Autodesk Inventor part; units mm, degrees
ref_plane "YZ Plane" through (0, 0, 0) normal (1, 0, 0) x (0, 1, 0)
ref_plane "XZ Plane" through (0, 0, 0) normal (0, 1, 0) x (-1, 0, 0)
ref_plane "XY Plane" through (0, 0, 0) normal (0, 0, 1) x (1, 0, 0)
sketch "Sketch1" plane through (0, 0, 0) normal (0, 1, 0) x (-1, 0, 0)
  line L0 (60, 25) -> (-60, 25)
  line L1 (-60, 25) -> (-60, -25)
  line L2 (-60, -25) -> (60, -25)
  line L3 (60, -25) -> (60, 25)
  point P0 (0, 0)
extrude "Extrusion1" add sketch "Sketch1" along normal mid plane 25
sketch "Sketch2" plane through (-60, 12.5, 25) normal (0, 0, 1) x (1, 0, 0)
  line L0 (0, -25) -> (120, -25)
  line L1 (60, -25) -> (20, -25)
  line L2 (20, -25) -> (20, -10)
  line L3 (20, -10) -> (100, -10)
  line L4 (100, -10) -> (100, -25)
  line L5 (100, -25) -> (60, -25)
  point P0 (60, -12.5)
  dimension "d5" = 15
  dimension "d6" = 80
extrude "Extrusion2" cut sketch "Sketch2" against normal through all
fillet "Fillet1" radius 12.5 2 edges at (60, 12.5, 0) (-60, 12.5, 0)
sketch "Sketch3" plane through (0, -12.5, 0) normal (0, -1, 0) x (1, 0, 0)
  line L0 (-60, 25) -> (-60, -25)
  line L1 (60, -25) -> (60, 25)
  point P0 (0, 0)
  point P1 (-50, 0)
  point P2 (50, 0)
hole "Hole1" at (-50, -12.5, 0) at (50, -12.5, 0) direction (0, 1, 0) diameter 3 depth 0.5 tip angle 118
properties part number "newsteelhandle" material "Steel"
Check sheet for the modelled part. Datum: model origin and axes. Units: mm. A direction names the side the tool comes from. Give positions to 0.01 mm unless a question says otherwise; leave off trailing zeros. Loops run counter-clockwise (first coordinate to the right, second up) from the corner with the lowest first, then second, coordinate; pieces in that order, holes last. Notation, with made-up numbers: M 34.5,-38 L 65.5,-38 A12 ccw 65.5,-24 Z; hole C -1,83.5 d8. An arc over 180 degrees is marked long. Return JSON: item names as keys, results as strings. Group by question number.
1. Mould release check, pull along X, two halves, no side actions. Record for faces 4 (the conical face through (50.078, -11.255, -0.248)), 5 (the cylindrical face through (56.241, 8.935, -0.35)), 6 (the flat face through (48, -12.5, 0)): released by +X, released by -X, zero draft, split by the parting line, or undercut.
2. Tool access check on faces 1 (the flat face through (-40, -5, 0)), 2 (the flat face through (60, -6, 0)), 3 (the cylindrical face through (51.464, -12.246, 0.325)). Record the directions out of +Z, -Z, +X, -X, +Y, -Y that give a thin tool (end or side, any length) a straight path to the whole face; none if there is none.
3. Cross-section at D-D on y = 7.75. Record the boundary of the cut face in (x, z), plus the area to 3 significant figures.
4. Cross-section at A-A on y = -2.75. Record the boundary of the cut face in (x, z), plus the area to 3 significant figures.
5. Go/stop test with flat-tipped pins: pin 1 (4 mm diameter, centred on x = 50, z = 0, fed in from +Y); pin 2 (1.8 mm diameter, centred on x = -50, z = 0, fed in from +Y); pin 3 (12 mm diameter, centred on y = 9, z = 2, fed in from +X). Record where each tip stops, or that it passes through.
6. Cross-section at C-C on x = -14. Record the boundary of the cut face in (y, z), plus the area to 3 significant figures.
7. Cross-section at B-B on z = -5.5. Record the boundary of the cut face in (x, y).
8. Thickness scan on L1, parallel to X at y = -12.3, z = 0; L2, parallel to Z at x = -50, y = -12.2; L3, parallel to X at y = -1.5, z = -22. Record the ranges inside material, lowest first.
Return value:
{
 "1": {"face 4": "undercut", "face 5": "released by +X", "face 6": "zero draft"},
 "2": {"face 1": "+Z, -Z, -Y", "face 2": "+Z, -Z, +X, +Y, -Y", "face 3": "-Y"},
 "3": {"outline": "M -57.31,-25 L 57.31,-25 L 57.31,25 L -57.31,25 Z", "area": "5,730 mm^2"},
 "4": {"outline": "M -60,-25 L -40,-25 L -40,25 L -60,25 Z; M 40,-25 L 60,-25 L 60,25 L 40,25 Z", "area": "2,000 mm^2"},
 "5": {"pin 1": "y = 12.49", "pin 2": "y = 12.4", "pin 3": "x = 59.63"},
 "6": {"outline": "M 2.5,-25 L 12.5,-25 L 12.5,25 L 2.5,25 Z", "area": "500 mm^2"},
 "7": {"outline": "M -60,-12.5 L -40,-12.5 L -40,2.5 L 40,2.5 L 40,-12.5 L 60,-12.5 L 60,0 A12.5 ccw 47.5,12.5 L -47.5,12.5 A12.5 ccw -60,0 Z"},
 "8": {"L1": "-60 to -51.5, -48.5 to -40, 40 to 48.5, 51.5 to 60", "L2": "-25 to -1.5, 1.5 to 25", "L3": "-60 to -40, 40 to 60"}
}
